from build123d import *

# Parameters (mm, degrees)
BOSS_EXTRUDE1_DEPTH = 33
BOSS_EXTRUDE2_DEPTH = 2
SKETCH3_W           = 29
SKETCH3_H           = 26.5
CUT_EXTRUDE1_DEPTH  = 2
SKETCH4_W           = 28.5
SKETCH4_H           = 25
CUT_EXTRUDE2_DEPTH  = 2


with BuildPart() as part:
    # Sketch1 → Boss-Extrude1 (new body)
    with BuildSketch(Plane(origin=(0, 0, 0), x_dir=(1, 0, 0), z_dir=(0, 1, 0))):
        Polygon((0, 0), (37.5, 0), (0, -37.5), align=None)
        Polygon((2, -2), (32.671572875, -2), (2, -32.671572875), align=None, mode=Mode.SUBTRACT)
    extrude(amount=BOSS_EXTRUDE1_DEPTH)

    # Sketch2 → Boss-Extrude2 (add)
    with BuildSketch(Plane.XZ):
        Polygon((2, 32.671572875), (32.671572875, 2), (2, 2), align=None)
    extrude(amount=-BOSS_EXTRUDE2_DEPTH)

    # Sketch3 → Cut-Extrude1 (cut)
    with BuildSketch(Plane(origin=(0, 0, 0), x_dir=(-1, 0, 0), z_dir=(0, 0, -1))):
        with Locations((-16.5, 16.25)):
            Rectangle(SKETCH3_W, SKETCH3_H)
    extrude(amount=-CUT_EXTRUDE1_DEPTH, mode=Mode.SUBTRACT)

    # Sketch4 → Cut-Extrude2 (cut)
    with BuildSketch(Plane.ZY):
        with Locations((18.75, 17.5)):
            Rectangle(SKETCH4_W, SKETCH4_H)
    extrude(amount=-CUT_EXTRUDE2_DEPTH, mode=Mode.SUBTRACT)


solid = part.part
Work out the finished part from the listing and answer in its coordinate system (mm). A direction names the side the tool comes from. Round coordinates to 2 decimals unless told otherwise and drop trailing zeros. Write each loop counter-clockwise with the first axis right and the second up, starting at its lowest first coordinate (ties: lowest second). Pieces come first, ordered by that corner, then holes. Notation, with made-up numbers: M 76,66 L 115,66 A15 ccw 115,84 Z; hole C 84,37.25 d4. An arc over 180 degrees is marked long. Use a Markdown table: item, result.
1) Which of the six approach directions +Z, -Z, +X, -X, +Y, -Y give full straight-line access (tool end or side, diameter ignored) to faces 1 (the face through (1, 17, 33)), 2 (the face through (17, 3, 1)), 3 (the face through (2, 17, 4)), 4 (the face through (11, 2, 11)), 5 (the face through (19, 16.3, 18.5))?
Taken from the geometry:
| item | result |
|---|---|
| face 1 | -X |
| face 2 | -Z |
| face 3 | none |
| face 4 | +Y |
| face 5 | +Z, +X, +Y, -Y |
2) The part is cut by section C-C on y = 30.5. Give the vertices of the cut face in (x, z).
Taken from the geometry:
| item | result |
|---|---|
| outline | M 0,0 L 37.5,0 L 0,37.5 Z; hole M 2,2 L 32.67,2 L 2,32.67 Z |
3) The part is cut by section D-D on y = 4.5. Give the vertices of the cut face in (x, z), plus the area to 3 significant figures.
Taken from the geometry:
| item | result |
|---|---|
| outline | M 0,0 L 2,0 L 2,32.67 L 32.67,2 L 31,2 L 31,0 L 37.5,0 L 0,37.5 Z |
| area | 175 mm2 |
4) Flat-ended cylindrical pins translate along their axes: pin 1 (3 mm diameter, centred on y = 9, z = 14, fed in from -X); pin 2 (12 mm diameter, centred on y = 9.5, z = 12, fed in from +X); pin 3 (10 mm diameter, centred on x = 10, y = 24, fed in from +Z). Find the tip coordinate at first contact, or state that the pin passes through.
Taken from the geometry:
| item | result |
|---|---|
| pin 1 | stops at x = 19.17 |
| pin 2 | stops at x = 31.5 |
| pin 3 | stops at z = 32.5 |
5) Determine the mould class of faces 6 (the face through (1, 17, 4.5)), 7 (the face through (0, 31, 19)), 8 (the face through (18, 31, 0)), 9 (the face through (20, 30, 2)) for opening direction Z: pulls with the +Z half, pulls with the -Z half, needs draft (parallel to the pull), parting line crosses it, or undercut.
Taken from the geometry:
| item | result |
|---|---|
| face 6 | undercut |
| face 7 | needs draft |
| face 8 | pulls with the -Z half |
| face 9 | undercut |
6) The part is cut by section A-A on y = 15. Give the vertices of the cut face in (x, z), plus the area to 3 significant figures.
Taken from the geometry:
| item | result |
|---|---|
| outline | M 0,0 L 2,0 L 2,4.5 L 0,4.5 Z; M 0,33 L 2,33 L 2,32.67 L 32.67,2 L 31,2 L 31,0 L 37.5,0 L 0,37.5 Z |
| area | 118 mm2 |
7) The part is cut by section B-B on x = 18. Give the vertices of the cut face in (y, z).
Taken from the geometry:
| item | result |
|---|---|
| outline | M 0,0 L 3,0 L 3,2 L 2,2 L 2,16.67 L 33,16.67 L 33,19.5 L 0,19.5 Z; M 29.5,0 L 33,0 L 33,2 L 29.5,2 Z |
8) Consider line 1 (Y direction, x = 4.5, z = 14); line 2 (X direction, y = 3.5, z = 33). Determine where each line is inside the solid, lowest interval first. Write a range as [from, to].
Taken from the geometry:
| item | result |
|---|---|
| line 1 | y = [0, 2] |
| line 2 | x = [0, 4.5] |
